```python
from build123d import *

# Parameters (mm, degrees)
F1_DEPTH = 25
F4_DEPTH = 69
F5_DEPTH = 25
F5_TAPER = -45


with BuildPart() as f1:
    # F0 (on Front) → F1 (new body)
    with BuildSketch(Plane.XZ):
        Polygon((-37.9215627909, 0), (-25.2369977534, 0), (-4.096057266, -27.3510906845), (10.9668616205, -27.3510906845), (10.9668616205, 0), (20.2160235494, 0), (20.2160235494, 10.7026007026), (11.2311234698, 10.7026007026), (11.495385319, 24.444213137), (-26.5543982792, 25.1759399431), (-26.5543982792, 12.0239099488), (-37.9215627909, 12.0239099488), align=None)
    extrude(amount=F1_DEPTH)


with BuildPart() as f4:
    # F3 (on Top) → F4 (new body)
    with BuildSketch(Plane.XY):
        Polygon((-24.5968098739, -9.0773625368), (-14.5968098739, -9.0773625368), (2.0060510084, -27.8395099328), (12.0059180895, -27.7879506378), (11.8940432243, -6.0899467872), (21.8940147673, -6.0660901471), (21.8623394592, 7.2112271297), (11.6888906335, 7.1869566299), (11.6327921873, 30.701704037), (-14.5968098739, 30.701704037), (-14.5968098739, 5.0683153725), (-24.5968098739, 5.0683153725), align=None)
    extrude(amount=F4_DEPTH)

    # F4_face (on face) → F5 (join)
    with BuildSketch(Plane(origin=(-0.7630345516, 3.1523470062, 0), x_dir=(1, 0, 0), z_dir=(0, 0, -1))):
        Polygon((12.3958267389, -27.5493570308), (12.4519251851, -4.0346096237), (22.6253740108, -4.0588801235), (22.6570493189, 9.2184371533), (12.6570777759, 9.2422937934), (12.768952641, 30.940297644), (2.76908556, 30.991856939), (-13.8337753223, 12.229709543), (-23.8337753223, 12.229709543), (-23.8337753223, -1.9159683663), (-13.8337753223, -1.9159683663), (-13.8337753223, -27.5493570308), align=None)
    extrude(amount=F5_DEPTH, taper=F5_TAPER)


solid = f4.part
```
Check sheet for the modelled part. Datum: model origin and axes. Units: mm. A direction names the side the tool comes from. Round coordinates to 2 decimals unless told otherwise and drop trailing zeros. Order: outer loops, then holes, each group sorted by start corner. A loop starts at its lowest first (then second) coordinate and runs counter-clockwise, first axis right, second up. Notation, with made-up numbers: (14, 0) -> (24, 0) arc R28 ccw to (24, 33) -> close; hole circle Ø1 at (64, -25). An arc over 180 degrees is marked (long way). One line per item, written item: value. Start each with the question number.
Q1. Gauge pin test, flat ends, axial feed: pin 1 Ø8 at (x, z) = (-17.5, 48) entering from -Y; pin 2 Ø1.5 at (y, z) = (-1, 52.5) entering from +X; pin 3 Ø11 at (x, z) = (-18, 38.5) entering from +Y. Record the tip position at first contact, or that the pin passes through.
Q2. Cross-section at A-A (z = 35). Record the boundary of the cut face in (x, y).
Q3. Thickness scan on line 1 (Y direction, x = 11, z = 48); line 2 (X direction, y = 16, z = 11); line 3 (Y direction, x = -20.5, z = 38). Record the ranges inside material, lowest first.
Q4. Set-up check for faces 1 (the face through (-1, 30.702, 34)), 2 (the face through (-6.41, -18.33, 34.02)), 3 (the face through (-14.597, 18, 34)), 4 (the face through (-24.597, -2, 34)): record each of +Z, -Z, +X, -X, +Y, -Y from which the full face is reachable in a straight line by a thin tool's end or side.
Completed:
1. pin 1: stops at y = -10.32
1. pin 2: stops at x = 21.88
1. pin 3: stops at y = 30.7
2. outline: (-24.6, -9.08) -> (-14.6, -9.08) -> (2.01, -27.84) -> (12.01, -27.79) -> (11.89, -6.09) -> (21.89, -6.07) -> (21.86, 7.21) -> (11.69, 7.19) -> (11.63, 30.7) -> (-14.6, 30.7) -> (-14.6, 5.07) -> (-24.6, 5.07) -> close
3. line 1: y = -27.79 to 30.7
3. line 2: x = -14.6 to 11.67
3. line 3: y = -9.08 to 5.07
4. face 1: +Z, +X, -X, +Y
4. face 2: +Z, -X, -Y
4. face 3: +Z, -X, +Y
4. face 4: +Z, -X, +Y, -Y
